```python
from build123d import *

# Parameters (mm, degrees)
SKETCH1_R           = 165.1
BOSS_EXTRUDE1_DEPTH = 6.35
SKETCH2_R           = 38.1
CUT_EXTRUDE1_DEPTH  = 6.35
CUT_EXTRUDE2_DEPTH  = 6.35


with BuildPart() as part:
    # Sketch1 → Boss-Extrude1 (new body)
    with BuildSketch(Plane(origin=(0, 0, 0), x_dir=(1, 0, 0), z_dir=(0, 1, 0))):
        with Locations(Location((0, 0, 0), (0, 0, 270))):
            Circle(SKETCH1_R)
    extrude(amount=BOSS_EXTRUDE1_DEPTH)

    # Sketch2 → Cut-Extrude1 (cut)
    with BuildSketch(Plane(origin=(0, 6.35, 0), x_dir=(1, 0, 0), z_dir=(0, 1, 0))):
        with Locations(Location((0, 0, 0), (0, 0, 270))):
            Circle(SKETCH2_R)
    extrude(amount=-CUT_EXTRUDE1_DEPTH, mode=Mode.SUBTRACT)

    # Sketch3 → Cut-Extrude2 (cut)
    with BuildSketch(Plane(origin=(0, 6.35, 0), x_dir=(1, 0, 0), z_dir=(0, 1, 0))):
        with BuildLine():
            Line((-33.02, -68.67400964), (-68.791666667, -143.070853416))
            ThreePointArc((-68.791666667, -143.070853416), (0, -158.75), (68.791666667, -143.070853416))
            Line((68.791666667, -143.070853416), (33.02, -68.67400964))
            ThreePointArc((33.02, -68.67400964), (0, -76.2), (-33.02, -68.67400964))
        make_face()
    extrude(amount=-CUT_EXTRUDE2_DEPTH, mode=Mode.SUBTRACT)


solid = part.part
```
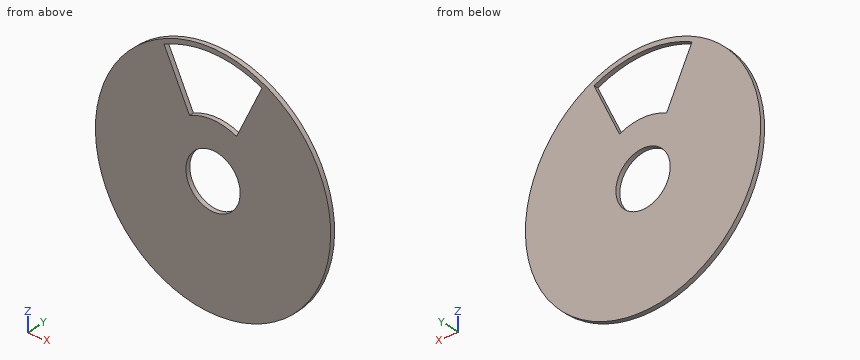
Geometry: final body of the model. Coordinates: model frame, mm. Round coordinates to 2 decimals unless told otherwise and drop trailing zeros. Order: outer loops, then holes, each group sorted by start corner. A loop starts at its lowest first (then second) coordinate and runs counter-clockwise, first axis right, second up. Notation, with made-up numbers: (75.5, 78) -> (107.5, 78) arc R29 cw to (107.5, 101) -> close; hole circle Ø7 at (29.5, 86). An arc over 180 degrees is marked (long way). Use one line per item in the form item = value. Start each with the question number.
1. Cut plane A-A (x = 0). Return the cut outline in (y, z).
2. Cut plane C-C (y = 1). Return the cut outline in (x, z), then the cut area to 3 significant figures.
3. Pin query (flat end, axial travel): pin 1 Ø1 at (x, y) = (99.5, 2.5) entering from -Z (3 decimals); pin 2 Ø3 at (x, y) = (17, 2) entering from -Z. Return the tip coordinate at first contact, or that it passes through.
4. Cut plane D-D (z = -104). Return the cut outline in (x, y), then the cut area to 3 significant figures.
5. Line query: probe 1 along X at (y, z) = (3.5, 0); probe 2 along Z at (x, y) = (13, 3.5); probe 3 along Z at (x, y) = (18.5, 0.5). Output: solid intervals per line, ascending.
6. Cut plane B-B (z = 0). Return the cut outline in (x, y).
Solution:
q1.outline = (0, -165.1) -> (6.35, -165.1) -> (6.35, -38.1) -> (0, -38.1) -> close; (0, 38.1) -> (6.35, 38.1) -> (6.35, 76.2) -> (0, 76.2) -> close; (0, 158.75) -> (6.35, 158.75) -> (6.35, 165.1) -> (0, 165.1) -> close
q2.outline = circle Ø330.2 at (0, 0); hole (-68.79, 143.07) -> (-33.02, 68.67) arc R76.2 cw to (33.02, 68.67) -> (68.79, 143.07) arc R158.75 ccw to start; hole circle Ø76.2 at (0, 0)
q2.area = 72,400 mm^2
q3.pin_1 = -132.125
q3.pin_2 = -164.37
q4.outline = (-128.23, 0) -> (128.23, 0) -> (128.23, 6.35) -> (-128.23, 6.35) -> close
q4.area = 1,630 mm^2
q5.probe_1 = -165.1 to -38.1, 38.1 to 165.1
q5.probe_2 = -164.59 to -35.81, 35.81 to 75.08, 158.22 to 164.59
q5.probe_3 = -164.06 to -33.31, 33.31 to 73.92, 157.67 to 164.06
q6.outline = (-165.1, 0) -> (-38.1, 0) -> (-38.1, 6.35) -> (-165.1, 6.35) -> close; (38.1, 0) -> (165.1, 0) -> (165.1, 6.35) -> (38.1, 6.35) -> close
